Here's the drawing with two shaded views (mm, measured from the low corner). I have some questions. A direction names the side the tool comes from. Round coordinates to 2 decimals unless told otherwise and drop trailing zeros. Write each loop counter-clockwise with the first axis right and the second up, starting at its lowest first coordinate (ties: lowest second). Pieces come first, ordered by that corner, then holes. Notation, with made-up numbers: M 0,35.25 L 21,35.25 A28 cw 21,60.25 Z; hole C 24.5,11.5 d2. An arc over 180 degrees is marked long. Answer as a JSON object with one key per item and string values. Group by question number.
1) Suppose I cut it at D-D, the plane z = 48.5. Write out the boundary of the cut face in (x, y).
2) On a 3-axis mill with a long thin cutter (end or side, diameter ignored), from which of +Z, -Z, +X, -X, +Y, -Y can I reach the whole of each face in a straight line? I mean the marked faces 1 and 2. Say none if no direction works.
3) Please list where these lines run through material, in increasing order: L1, parallel to Y at x = 28, z = 2 (1 decimal); L2, parallel to Z at x = 14.5, y = 6; L3, parallel to Y at x = 8.5, z = 2.3. Write a range as [from, to].
4) Suppose I cut it at B-B, the plane z = 23. Write out the boundary of the cut face in (x, y).
5) Suppose I cut it at A-A, the plane y = 22. Write out the boundary of the cut face in (x, z), and give its area (3 significant figures).
6) I'm going to push flat-ended pins straight in: pin 1 Ø3 at (y, z) = (5.5, 17.58) entering from +X; pin 2 Ø13.5 at (y, z) = (17.5, 29.58) entering from +X; pin 3 Ø17 at (x, y) = (20.5, 23) entering from +Z. Where does each tip first touch, or does it pass through?
7) Suppose I cut it at C-C, the plane x = 28.75. Write out the boundary of the cut face in (y, z) (1 decimal).
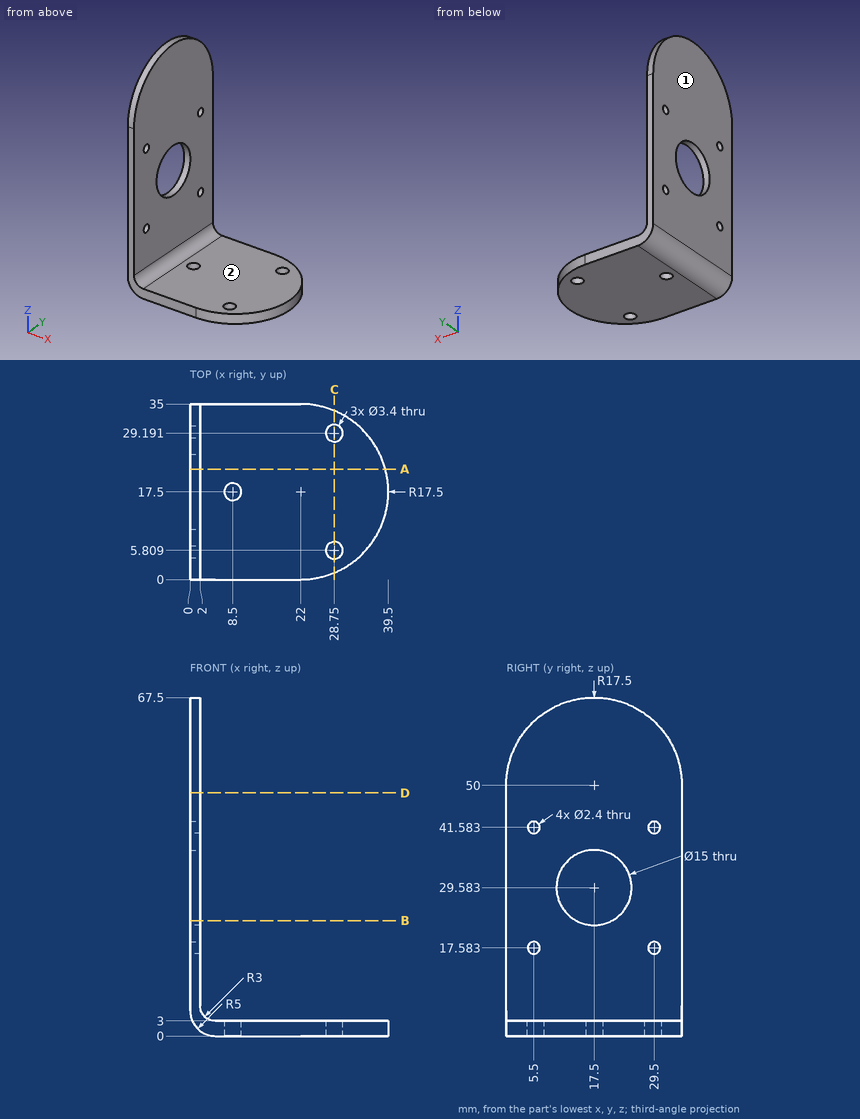
Results:
{
 "1": {"outline": "M 0,0 L 2,0 L 2,35 L 0,35 Z"},
 "2": {"face 1": "+Z, -Z, -X, +Y, -Y", "face 2": "+Z, +X, +Y, -Y"},
 "3": {"L1": "[1.1, 4.3], [7.3, 27.7], [30.7, 33.9]", "L2": "[0, 3]", "L3": "[0, 15.8], [19.2, 35]"},
 "4": {"outline": "M 0,0 L 2,0 L 2,13.91 L 0,13.91 Z; M 0,21.09 L 2,21.09 L 2,35 L 0,35 Z"},
 "5": {"outline": "M 0,5 A5 ccw 5,0 L 38.91,0 L 38.91,3 L 5,3 A3 cw 2,6 L 2,23.58 L 0,23.58 Z; M 0,35.58 L 2,35.58 L 2,66.91 L 0,66.91 Z", "area": "217 mm^2"},
 "6": {"pin 1": "x = 2", "pin 2": "through", "pin 3": "z = 3"},
 "7": {"outline": "M 1.4,0 L 4.1,0 L 4.1,3 L 1.4,3 Z; M 7.5,0 L 27.5,0 L 27.5,3 L 7.5,3 Z; M 30.9,0 L 33.6,0 L 33.6,3 L 30.9,3 Z"}
}
